Geometry check sheet. Reference: the model listing, model coordinates, mm. A direction names the side the tool comes from. Give positions to 0.01 mm unless a question says otherwise; leave off trailing zeros. Order: outer loops, then holes, each group sorted by start corner. A loop starts at its lowest first (then second) coordinate and runs counter-clockwise, first axis right, second up. Notation, with made-up numbers: M 30,35 L 40,35 A16 cw 40,49 Z; hole C -38.5,35.5 d11. An arc over 180 degrees is marked long. Answer as CSV lines item,"result". Start each with the question number.
Q1. Thickness scan on line 1 (X direction, y = -0.5, z = 0); line 2 (Y direction, x = -5.5, z = -1.25); line 3 (X direction, y = -2.6, z = -0.2). Record the ranges inside material, lowest first.
Q2. Set-up check for faces 1 (the cylindrical face through (9.45, 1.06, -1.43)), 2 (the cylindrical face through (-2.052, -2.739, -0.108)), 3 (the cylindrical face through (-9.45, -1.51, 1.43)): record each of +Z, -Z, +X, -X, +Y, -Y from which the full face is reachable in a straight line by a thin tool's end or side.
Q3. Section check C-C, the plane x = 2.54. Record the boundary of the cut face in (y, z), then the cut area to 3 significant figures.
Q4. Section check A-A, the plane y = -0.65. Count the separate pieces of the cut face and the enclosed holes in it, then the cut area to 3 significant figures.
Q5. Go/stop test with flat-tipped pins: pin 1 (2 mm diameter, centred on x = 9.5, z = 0.5, fed in from -Y); pin 2 (1.5 mm diameter, centred on y = 0, z = -1.5, fed in from +X); pin 3 (2 mm diameter, centred on y = 0.5, z = -1, fed in from +X); pin 4 (1.4 mm diameter, centred on x = 11.5, z = 0, fed in from +Y). Record where each tip stops, or that it passes through.
Q6. Mould release check, pull along X, two halves, no side actions. Record for faces 4 (the cylindrical face through (-4.592, -2.739, -0.108)), 5 (the cylindrical face through (12.35, -0.51, 1.43)), 6 (the flat face through (0, -3.5, 0)): +X half, -X half, draft (parallel to the pull), parting line (faces both ways), or undercut.
Q7. Section check B-B, the plane x = 11.5. Record the boundary of the cut face in (y, z), then the cut area to 3 significant figures.
```python
from build123d import *

# Parameters (mm, degrees)
SKETCH_1_W          = 20.1
SKETCH_1_H          = 4
EXTRUDE_1_DEPTH     = 2.1
SKETCH_1_3_W        = 25.9
SKETCH_1_3_H        = 4
EXTRUDE_2_DEPTH     = 1
EXTRUDE_START       = -1
SKETCH_1_4_W        = 20.1
SKETCH_1_4_H        = 4
EXTRUDE_4_DEPTH     = 1
FILLET_2_R          = 2
FILLET_1_R          = 2
SKETCH_2_R          = 0.75
CUT_EXTRUDE_1_DEPTH = 14.465233009
EXTRUDE_START_2     = -3.1
SKETCH_3_R          = 0.5
EXTRUDE_3_DEPTH     = 5.6


with BuildPart() as part:
    # 草图1 → 凸台-拉伸1 (new body)
    with BuildSketch(Plane(origin=(0, 0, 0), x_dir=(1, 0, 0), z_dir=(0, 1, 0))):
        Rectangle(SKETCH_1_W, SKETCH_1_H)
    extrude(amount=EXTRUDE_1_DEPTH)

    # 草图1<3> → 凸台-拉伸2 (add)
    with BuildSketch(Plane(origin=(0, 0, 0), x_dir=(1, 0, 0), z_dir=(0, 1, 0))):
        Rectangle(SKETCH_1_3_W, SKETCH_1_3_H)
    extrude(amount=-EXTRUDE_2_DEPTH)

    # 草图1<4> → 凸台-拉伸4 (add)
    with BuildSketch(Plane(origin=(0, 0, 0), x_dir=(1, 0, 0), z_dir=(0, 1, 0)).offset(EXTRUDE_START)):
        Rectangle(SKETCH_1_4_W, SKETCH_1_4_H)
    extrude(amount=-EXTRUDE_4_DEPTH)

    # 圆角2
    fillet_2_edges = [part.edges().sort_by_distance(p)[0] for p in [
        (12.95, -0.5, 2),
        (12.95, -0.5, -2),
        (-12.95, -0.5, 2),
        (-12.95, -0.5, -2),
    ]]
    fillet(fillet_2_edges, radius=FILLET_2_R - 0.0001)  # a hair under: the kernel refuses the full size

    # 圆角1
    fillet_1_edges = [part.edges().sort_by_distance(p)[0] for p in [
        (10.05, 1.05, -2),
        (10.05, 1.05, 2),
        (-10.05, 1.05, 2),
        (-10.05, 1.05, -2),
        (-10.05, -1.5, -2),
        (-10.05, -1.5, 2),
        (10.05, -1.5, 2),
        (10.05, -1.5, -2),
    ]]
    fillet(fillet_1_edges, radius=FILLET_1_R - 0.0001)  # a hair under: the kernel refuses the full size

    # 草图2 → 切除-拉伸1 (cut, through all)
    with BuildSketch(Plane(origin=(0, -1, 0), x_dir=(-1, 0, 0), z_dir=(0, -1, 0))):
        with Locations(Location((11.5, 0, 0), (0, 0, 90))):
            Circle(SKETCH_2_R)
        with Locations(Location((-11.5, 0, 0), (0, 0, 90))):
            Circle(SKETCH_2_R)
    extrude(amount=-CUT_EXTRUDE_1_DEPTH, mode=Mode.SUBTRACT)

    # 草图3 → 凸台-拉伸3 (add)
    with BuildSketch(Plane.XZ.offset(1).offset(EXTRUDE_START_2)):
        with Locations(Location((0, 0, 0), (0, 0, 90))):
            Circle(SKETCH_3_R)
        with Locations(Location((2.54, 0, 0), (0, 0, 90))):
            Circle(SKETCH_3_R)
        with Locations(Location((-2.54, 0, 0), (0, 0, 90))):
            Circle(SKETCH_3_R)
        with Locations(Location((-5.08, 0, 0), (0, 0, 90))):
            Circle(SKETCH_3_R)
        with Locations(Location((5.08, 0, 0), (0, 0, 90))):
            Circle(SKETCH_3_R)
    extrude(amount=EXTRUDE_3_DEPTH)


solid = part.part
```
Answer block:
1,line 1,"x = -12.95 to -12.25, -10.75 to 10.75, 12.25 to 12.95"
1,line 2,"y = -2 to 2.1"
1,line 3,"x = -5.54 to -4.62, -3 to -2.08, -0.46 to 0.46, 2.08 to 3, 4.62 to 5.54"
2,face 1,"-Z, +X, +Y"
2,face 2,"-Y"
2,face 3,"+Z, -X, -Y"
3,outline,"M -3.5,-0.5 L -2,-0.5 L -2,-2 L 2.1,-2 L 2.1,2 L -2,2 L -2,0.5 L -3.5,0.5 Z"
3,area,"17.9 mm2"
4,separate pieces,"1"
4,enclosed holes,"2"
4,area,"96.6 mm2"
5,pin 1,"stops at y = -2"
5,pin 2,"stops at x = 12.8"
5,pin 3,"stops at x = 12.95"
5,pin 4,"passes through"
6,face 4,"undercut"
6,face 5,"+X half"
6,face 6,"draft"
7,outline,"M -1,-1.92 L 0,-1.92 L 0,-0.75 L -1,-0.75 Z; M -1,0.75 L 0,0.75 L 0,1.92 L -1,1.92 Z"
7,area,"2.35 mm2"
